from build123d import *

# Parameters (mm, degrees)
PAD007_DEPTH            = 1
SKETCH014_R             = 4
PAD008_DEPTH            = 2.5
HOLE_D                  = 3.6
HOLE_DEPTH              = 25
HOLE_CSINK_D            = 6.7
HOLE_CSINK_ANGLE        = 90
BODY003_PLACEMENT_ANGLE = 180


with BuildPart() as part:
    # Sketch013 → Pad007 (new body)
    with BuildSketch(Plane.XY):
        with BuildLine():
            ThreePointArc((-40, 29), (-42.828427, 27.828427), (-44, 25))
            Line((-44, -25), (-44, 25))
            ThreePointArc((-44, -25), (-42.828427, -27.828427), (-40, -29))
            Line((40, -29), (-40, -29))
            ThreePointArc((40, -29), (42.828427, -27.828427), (44, -25))
            Line((44, 25), (44, -25))
            ThreePointArc((44, 25), (42.828427, 27.828427), (40, 29))
            Line((-40, 29), (40, 29))
        make_face()
    extrude(amount=PAD007_DEPTH)

    # Sketch014 → Pad008 (join)
    with BuildSketch(Plane.XY):
        with Locations((-40, 25)):
            Circle(SKETCH014_R)
        with Locations((18, 25)):
            Circle(SKETCH014_R)
        with Locations((40, 25)):
            Circle(SKETCH014_R)
        with Locations((40, -25)):
            Circle(SKETCH014_R)
        with Locations((18, -25)):
            Circle(SKETCH014_R)
        with Locations((-40, -25)):
            Circle(SKETCH014_R)
    extrude(amount=PAD008_DEPTH)

    # Hole
    with Locations(Plane(origin=(0, 0, 0), x_dir=(1, 0, 0), z_dir=(0, 0, -1))):
        with Locations((-40, -25), (18, -25), (40, -25), (40, 25), (18, 25), (-40, 25)):
            CounterSinkHole(HOLE_D / 2, HOLE_CSINK_D / 2, depth=HOLE_DEPTH, counter_sink_angle=HOLE_CSINK_ANGLE)


with BuildPart() as part_1:
    # Body003 placement: moved
    add(part.part.moved(Location((0, 0, 133.1))).rotate(Axis((0, 0, 133.1), (0, 1, 0)), BODY003_PLACEMENT_ANGLE))


solid = part_1.part
Can you work these out from the model? Positions are in its coordinate system, mm. A direction names the side the tool comes from. Give positions to 0.01 mm unless a question says otherwise; leave off trailing zeros. Write each loop counter-clockwise with the first axis right and the second up, starting at its lowest first coordinate (ties: lowest second). Pieces come first, ordered by that corner, then holes. Notation, with made-up numbers: M 39,39.25 L 64,39.25 A12 cw 64,58.25 Z; hole C 20,-22.5 d11. An arc over 180 degrees is marked long. Answer in a Markdown table with one row per item. Add a question column.
Item 1: Please list where these lines run through material, in increasing order: L1, parallel to Y at x = 40, z = 131.15; L2, parallel to X at y = 25, z = 131.3; L3, parallel to X at y = -23.5, z = 132.05.
Item 2: For pin 1 Ø10 at (x, y) = (29, 2) entering from -Z; pin 2 Ø3 at (x, y) = (-40, -25) entering from +Z; pin 3 Ø6 at (x, y) = (40, -25) entering from +Z; pin 4 Ø4 at (x, y) = (-18, -25) entering from +Z, each with a flat end and sliding along its axis, tell me the tip position at first contact or that it passes through.
Item 3: On a 3-axis mill with a long thin cutter (end or side, diameter ignored), from which of +Z, -Z, +X, -X, +Y, -Y can I reach the whole of each face in a straight line? I mean faces 3 (the cylindrical face through (-39.032, 23.482, 131.068)), 4 (the cylindrical face through (-15.05, -22.3, 131.36)). Say none if no direction works.
Item 4: Imagine slicing it at B-B, the plane y = 14. Write out the boundary of the cut face in (x, z), plus the area to 3 significant figures.
Item 5: We'd pull the mould along Y, two halves only. Please class faces 1 (the cylindrical face through (-17.479, 28.966, 131.36)), 2 (the flat face through (-42, 24, 130.6)): released by +Y, released by -Y, zero draft, split by the parting line, or undercut.
Item 6: Imagine slicing it at C-C, the plane x = -12. Write out the boundary of the cut face in (y, z), plus the area to 3 significant figures.
Item 7: Imagine slicing it at A-A, the plane z = 132.65. Write out the boundary of the cut face in (x, y).
Evaluation:
| question | item | result |
|---|---|---|
| 1 | L1 | y = -29 to -26.8, -23.2 to -21, 21 to 23.2, 26.8 to 29 |
| 1 | L2 | x = -44 to -41.8, -38.2 to -36, -22 to -19.8, -16.2 to -14, 36 to 38.2, 41.8 to 44 |
| 1 | L3 | x = -43.71 to -41.74, -38.26 to -36.29, -21.71 to -19.74, -16.26 to -14.29, 36.29 to 38.26, 41.74 to 43.71 |
| 2 | pin 1 | stops at z = 132.1 |
| 2 | pin 2 | passes through |
| 2 | pin 3 | stops at z = 132.75 |
| 2 | pin 4 | stops at z = 131.75 |
| 3 | face 3 | +Z, -Z |
| 3 | face 4 | -Z |
| 4 | outline | M -44,132.1 L 44,132.1 L 44,133.1 L -44,133.1 Z |
| 4 | area | 88.0 mm² |
| 5 | face 1 | undercut |
| 5 | face 2 | zero draft |
| 6 | outline | M -29,132.1 L 29,132.1 L 29,133.1 L -29,133.1 Z |
| 6 | area | 58.0 mm² |
| 7 | outline | M -44,-25 A4 ccw -40,-29 L 40,-29 A4 ccw 44,-25 L 44,25 A4 ccw 40,29 L -40,29 A4 ccw -44,25 Z; hole C -40,-25 d5.8; hole C -40,25 d5.8; hole C -18,-25 d5.8; hole C -18,25 d5.8; hole C 40,-25 d5.8; hole C 40,25 d5.8 |
